Could you check a few things on this model? Use its own coordinates, in mm. A direction names the side the tool comes from. Give positions to 0.01 mm unless a question says otherwise; leave off trailing zeros. Loops run counter-clockwise (first coordinate to the right, second up) from the corner with the lowest first, then second, coordinate; pieces in that order, holes last. Notation, with made-up numbers: (17, 39.5) -> (29, 39.5) arc R19 cw to (29, 68.5) -> close; hole circle Ø8 at (5, 50.25). An arc over 180 degrees is marked (long way). Write item = value, one per line. Start each with the question number.
1) I want a section at A-A (x = 1.5). List the corners of the cut face in (y, z) for me, and give its area (3 significant figures).
2) If we mould it in two halves opening along Z, with no side actions, what happens to faces 5 (the face through (9, 0, -6)), 6 (the face through (1, 1, -8)), 7 (the face through (18, 1, -8))? For each: +Z half, -Z half, draft (parallel to the pull), parting line (faces both ways), or undercut.
3) I need wall thicknesses on probe 1 along Z at (x, y) = (1, 0.5); probe 2 along X at (y, z) = (0.45, -4.75); probe 3 along Z at (x, y) = (15, 0.5). Which ranges of each line are inside material? Lowest first, please. Write a range as from..to.
4) I'm going to push flat-ended pins straight in: pin 1 Ø0.6 at (x, y) = (0.5, 1) entering from -Z; pin 2 Ø1.5 at (x, z) = (8.5, -13.5) entering from -Y. Where does each tip first touch, or does it pass through?
5) I want a section at D-D (z = -11). List the corners of the cut face in (x, y) for me.
6) I want a section at C-C (x = -18.5). List the corners of the cut face in (y, z) for me, and give its area (3 significant figures).
7) On a 3-axis mill with a long thin cutter (end or side, diameter ignored), from which of +Z, -Z, +X, -X, +Y, -Y can I reach the whole of each face in a straight line? I mean faces 1 (the face through (10, 0.55, -13)), 2 (the face through (-11.804, 0.608, -9.988)), 3 (the face through (17, 1, -10)), 4 (the face through (10, 1.3, -13)). Say none if no direction works.
8) I want a section at B-B (z = -3.25). List the corners of the cut face in (x, y) for me.
from build123d import *

# Parameters (mm, degrees)
AUFSATZ_LINEAR_AUSTRAGEN1_DEPTH = 1.9
SKIZZE4_R                       = 0.5
AUFSATZ_LINEAR_AUSTRAGEN3_DEPTH = 28
SKIZZE5_W                       = 1.322669318
SKIZZE5_H                       = 0.6
SKIZZE5_H_2                     = 0.55
SCHNITT_LINEAR_AUSTRAGEN1_DEPTH = 16


with BuildPart() as part:
    # Skizze1 → Aufsatz-Linear austragen1 (new body)
    with BuildSketch(Plane(origin=(0, 0, 0), x_dir=(1, 0, 0), z_dir=(0, 1, 0))):
        Polygon((0, 0), (19, 0), (19, 8), (17, 8), (17, 14), (2, 14), (2, 8), (0, 8), align=None)
    extrude(amount=AUFSATZ_LINEAR_AUSTRAGEN1_DEPTH)

    # Skizze4 → Aufsatz-Linear austragen3 (add)
    with BuildSketch(Plane.ZY.offset(-2)):
        with Locations(Location((-9.5, 0.5, 0), (0, 0, 270))):
            Circle(SKIZZE4_R)
    extrude(amount=AUFSATZ_LINEAR_AUSTRAGEN3_DEPTH)

    # Skizze5 → Schnitt-Linear austragen1 (cut)
    with BuildSketch(Plane(origin=(17, 0, 0), x_dir=(0, 0, -1), z_dir=(1, 0, 0))):
        with Locations((13.338665341, 1.6)):
            Rectangle(SKIZZE5_W, SKIZZE5_H)
        with Locations((13.338665341, 0.275)):
            Rectangle(SKIZZE5_W, SKIZZE5_H_2)
    extrude(amount=-SCHNITT_LINEAR_AUSTRAGEN1_DEPTH, mode=Mode.SUBTRACT)


solid = part.part
Answer list:
q1.outline = circle Ø1 at (0.5, -9.5); (0, -8) -> (1.9, -8) -> (1.9, 0) -> (0, 0) -> close
q1.area = 16.0 mm^2
q2.face_5 = draft
q2.face_6 = undercut
q2.face_7 = -Z half
q3.probe_1 = -10..-9, -8..0
q3.probe_2 = 0..19
q3.probe_3 = -12.68..0
q4.pin_1 = -9.96
q4.pin_2 = 0.55
q5.outline = (2, 0) -> (17, 0) -> (17, 1.9) -> (2, 1.9) -> close
q6.outline = circle Ø1 at (0.5, -9.5)
q6.area = 0.785 mm^2
q7.face_1 = -Z, +X, -X, -Y
q7.face_2 = -X
q7.face_3 = -Z, +X, +Y, -Y
q7.face_4 = -Z, +X, -X, +Y
q8.outline = (0, 0) -> (19, 0) -> (19, 1.9) -> (0, 1.9) -> close
